Source: CAD feature listing. Evaluate the final solid. Frame: model axes, mm. A direction names the side the tool comes from. Give positions to 0.01 mm unless a question says otherwise; leave off trailing zeros. Order: outer loops, then holes, each group sorted by start corner. A loop starts at its lowest first (then second) coordinate and runs counter-clockwise, first axis right, second up. Notation, with made-up numbers: M -15.75,66.25 L 38.25,66.25 A12 ccw 38.25,84.25 Z; hole C 80,86.5 d1. An arc over 180 degrees is marked long. Answer as a JSON object with one key per item and string values. Group by question number.
1. Pin query (flat end, axial travel): P1, Ø2.5, axis at x = 0.5, y = 9.5, coming from the +Z side; P2, Ø4, axis at y = -8, z = 25.5, coming from the +X side; P3, Ø4, axis at x = -7, z = 37.5, coming from the +Y side (3 decimals); P4, Ø4, axis at y = -9, z = 9.5, coming from the -X side. Return the tip coordinate at first contact, or that it passes through.
2. Material intervals for L1, parallel to Y at x = 0, z = 31.5; L2, parallel to Z at x = 3.5, y = -7.25; L3, parallel to Z at x = 3.75, y = 3.5, sorted ascending. Write a range as [from, to].
3. Section query B-B (z = 37). Output: boundary loops of the cut face in (x, y), plus the area to 3 significant figures.
4. Set-up query: faces 1 (the flat face through (0, -10, 28.4)), 2 (the flat face through (0, 0, 54.2)), 3 (the flat face through (0, 2.4, 42.2)). Return all of +Z, -Z, +X, -X, +Y, -Y with unobstructed straight access to the full face (end or side cutting, diameter ignored); none if empty.
5. Pull-direction query (X, two-part tool) for faces 4 (the flat face through (0, 0, 0)), 5 (the cylindrical face through (8.5, 0.07, 30.94)), 6 (the cylindrical face through (-7.493, 0.33, 34.14)); classes: +X half, -X half, draft (parallel to the pull), parting line (faces both ways), or undercut.
6. Section query A-A (x = 0). Output: boundary loops of the cut face in (y, z), plus the area to 3 significant figures.
from build123d import *

# Parameters (mm, degrees)
ESQUISSE1_R             = 13
BOSS_EXTRU_1_DEPTH      = 33.4
ESQUISSE2_R             = 7.5
BOSS_EXTRU_2_DEPTH      = 2
ESQUISSE3_R             = 3
BOSS_EXTRU_3_DEPTH      = 18.8
ENL_V_START             = -12
ENL_V_MAT_EXTRU_1_DEPTH = 12
CHANFREIN1_SIZE         = 0.5
ESQUISSE5_R             = 1.5
ENL_V_MAT_EXTRU_2_DEPTH = 5
CONG_1_R                = 0.5


with BuildPart() as part:
    # Esquisse1 → Boss.-Extru.1 (new body)
    with BuildSketch(Plane.XY):
        Circle(ESQUISSE1_R)
    extrude(amount=BOSS_EXTRU_1_DEPTH)

    # Esquisse2 → Boss.-Extru.2 (add)
    with BuildSketch(Plane.XY.offset(33.4)):
        Circle(ESQUISSE2_R)
    extrude(amount=BOSS_EXTRU_2_DEPTH)

    # Esquisse3 → Boss.-Extru.3 (add)
    with BuildSketch(Plane.XY.offset(35.4)):
        Circle(ESQUISSE3_R)
    extrude(amount=BOSS_EXTRU_3_DEPTH)

    # Esquisse4 → Enlèv. mat.-Extru.1 (cut)
    with BuildSketch(Plane.XY.offset(54.2).offset(ENL_V_START)):
        with BuildLine():
            Line((-2.236067977, 2), (2.236067977, 2))
            ThreePointArc((2.236067977, 2), (0, 3), (-2.236067977, 2))
        make_face()
    extrude(amount=ENL_V_MAT_EXTRU_1_DEPTH, mode=Mode.SUBTRACT)

    # Chanfrein1
    chanfrein1_edges = [part.edges().sort_by_distance(p)[0] for p in [
        (-1.070466269, -2.802517077, 54.2),
        (0, 2, 54.2),
        (-7.5, 0, 35.4),
    ]]
    chamfer(chanfrein1_edges, length=CHANFREIN1_SIZE)

    # Esquisse5 → Enlèv. mat.-Extru.2 (cut)
    with BuildSketch(Plane.XY.offset(33.4)):
        with Locations((0, 10)):
            Circle(ESQUISSE5_R)
        with Locations((10, 0)):
            Circle(ESQUISSE5_R)
        with Locations((0, -10)):
            Circle(ESQUISSE5_R)
        with Locations((-10, 0)):
            Circle(ESQUISSE5_R)
    extrude(amount=-ENL_V_MAT_EXTRU_2_DEPTH, mode=Mode.SUBTRACT)

    # Congé1
    cong_1_edges = [part.edges().sort_by_distance(p)[0] for p in [
        (-13, 0, 33.4),
    ]]
    fillet(cong_1_edges, radius=CONG_1_R)


solid = part.part
Answer sheet:
{
 "1": {"P1": "z = 33.4", "P2": "x = 11.53", "P3": "through", "P4": "x = -10.95"},
 "2": {"L1": "[-13, -11.5], [-8.5, 8.5], [11.5, 13]", "L2": "[0, 33.4]", "L3": "[0, 35.4]"},
 "3": {"outline": "C 0,0 d6", "area": "28.3 mm^2"},
 "4": {"face 1": "+Z", "face 2": "+Z, +X, -X, +Y, -Y", "face 3": "+Z, +X, -X, +Y"},
 "5": {"face 4": "draft", "face 5": "undercut", "face 6": "parting line"},
 "6": {"outline": "M -13,0 L 13,0 L 13,32.9 A0.5 ccw 12.5,33.4 L 11.5,33.4 L 11.5,28.4 L 8.5,28.4 L 8.5,33.4 L 7.5,33.4 L 7.5,34.9 L 7,35.4 L 3,35.4 L 3,42.2 L 2,42.2 L 2,53.7 L 1.5,54.2 L -2.5,54.2 L -3,53.7 L -3,35.4 L -7,35.4 L -7.5,34.9 L -7.5,33.4 L -8.5,33.4 L -8.5,28.4 L -11.5,28.4 L -11.5,33.4 L -12.5,33.4 A0.5 ccw -13,32.9 Z", "area": "969 mm^2"}
}
